Autodesk Inventor part; units mm, degrees
ref_plane "XY Plane" through (0, 0, 0) normal (0, 0, 1) x (1, 0, 0)
sketch "Sketch3" plane through (0, 0, 0) normal (0, 0, 1) x (1, 0, 0)
  circle A0 centre (0, 0) radius 7.62
  dimension "d3" = 15.24
extrude "Extrusion2" add sketch "Sketch3" along normal blind 1.27
sketch "Sketch4" plane through (0, 0, 1.27) normal (0, 0, 1) x (1, 0, 0)
  line L0 (0, 7.5994) -> (6.5813, 3.7997)
  line L1 (6.5813, 3.7997) -> (6.5813, -3.7997)
  line L2 (6.5813, -3.7997) -> (0, -7.5994)
  line L3 (0, -7.5994) -> (-6.5813, -3.7997)
  line L4 (-6.5813, -3.7997) -> (-6.5813, 3.7997)
  line L5 (-6.5813, 3.7997) -> (0, 7.5994)
  point P0 (0, 0)
  point P1 (0, 0)
extrude "Extrusion3" add sketch "Sketch4" along normal blind 18.034
sketch "Sketch5" plane through (0, 0, 19.304) normal (0, 0, 1) x (1, 0, 0)
  circle A0 centre (0, 0) radius 6.35
  dimension "d8" = 12.7
extrude "Extrusion4" add sketch "Sketch5" along normal blind 1.27
sketch "Sketch6" plane through (0, 0, 20.574) normal (0, 0, 1) x (1, 0, 0)
  circle A0 centre (0, 0) radius 6.35
  line L0 (6.5813, 3.7997) -> (6.5813, -3.7997)
  line L1 (6.5813, -3.7997) -> (0, -7.5994)
  line L2 (0, -7.5994) -> (-6.5813, -3.7997)
  line L3 (-6.5813, -3.7997) -> (-6.5813, 3.7997)
  line L4 (-6.5813, 3.7997) -> (0, 7.5994)
  line L5 (0, 7.5994) -> (6.5813, 3.7997)
  circle A1 centre (0, 0) radius 7.62
  line L6 (0, 7.5994) -> (6.5813, 3.7997)
  line L7 (6.35, 3.6662) -> (6.35, -3.6662)
  line L8 (6.35, -3.6662) -> (0, -7.3323)
  line L9 (0, -7.3323) -> (-6.35, -3.6662)
  line L10 (-6.35, -3.6662) -> (-6.35, 3.6662)
  line L11 (-6.35, 3.6662) -> (0, 7.3323)
  line L12 (0, 7.3323) -> (6.35, 3.6662)
  point P0 (3.175, 5.4993)
extrude "Extrusion5" add sketch "Sketch6" along normal blind 1.27 contours A0 | L7 L8 A0 | A0 L12 L7 | A0 L11 L12 | L8 L9 A0 | A0 L10 L11 | L9 L10 A0
sketch "Sketch7" plane through (0, 0, 21.844) normal (0, 0, 1) x (1, 0, 0)
  circle A0 centre (0, 0) radius 3
  dimension "d13" = 6
extrude "Extrusion6" cut sketch "Sketch7" against normal up to next
ref_plane "Work Plane1" through (0, 0, 0) normal (0, 1, 0) x (-1, 0, 0)
ref_plane "Work Plane2" through (0, 0, 0) normal (1, 0, 0) x (0, 1, 0)
properties part number "BaneBots-T40-6mm-Shaft-Adapter"
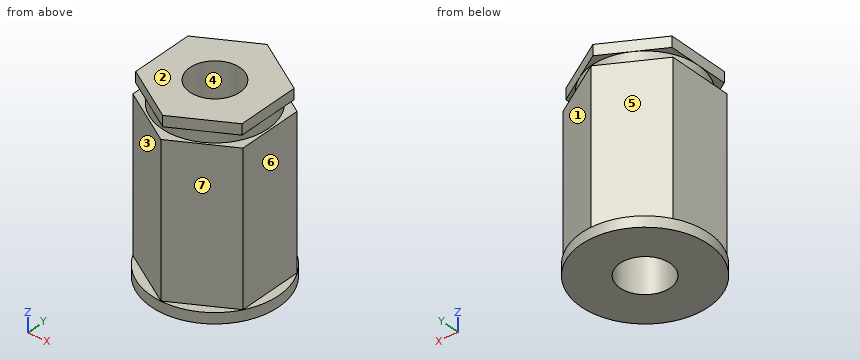
Geometry check sheet. Reference: the model listing, model coordinates, mm. Face numbers are marked on the shaded views. A direction names the side the tool comes from. Give positions to 0.01 mm unless a question says otherwise; leave off trailing zeros. Write each loop counter-clockwise with the first axis right and the second up, starting at its lowest first coordinate (ties: lowest second). Pieces come first, ordered by that corner, then holes. Notation, with made-up numbers: (56.25, 55) -> (78.25, 55) arc R16 ccw to (78.25, 77) -> close; hole circle Ø2 at (-31, 54). An arc over 180 degrees is marked (long way). Use one line per item in the form item = value.
Item 1: Sectioned sample at D-D on y = 5. Enter the section's corners in (x, z).
Results list:
outline = (-5.75, 0) -> (5.75, 0) -> (5.75, 1.27) -> (4.5, 1.27) -> (4.5, 19.3) -> (3.91, 19.3) -> (3.91, 20.57) -> (4.04, 20.57) -> (4.04, 21.84) -> (-4.04, 21.84) -> (-4.04, 20.57) -> (-3.91, 20.57) -> (-3.91, 19.3) -> (-4.5, 19.3) -> (-4.5, 1.27) -> (-5.75, 1.27) -> close
Item 2: Sectioned sample at B-B on y = -1.5. Enter the section's corners in (x, z).
Results list:
outline = (-7.47, 0) -> (-2.6, 0) -> (-2.6, 21.84) -> (-6.35, 21.84) -> (-6.35, 20.57) -> (-6.17, 20.57) -> (-6.17, 19.3) -> (-6.58, 19.3) -> (-6.58, 1.27) -> (-7.47, 1.27) -> close; (2.6, 0) -> (7.47, 0) -> (7.47, 1.27) -> (6.58, 1.27) -> (6.58, 19.3) -> (6.17, 19.3) -> (6.17, 20.57) -> (6.35, 20.57) -> (6.35, 21.84) -> (2.6, 21.84) -> close
Item 3: Access from +Z, -Z, +X, -X, +Y, -Y to the whole of each face (thin tool, end or side, straight path). Record for the marked faces 5, 6 and 7.
Results list:
face_5 = +Z, -X, +Y
face_6 = +Z, +X, +Y, -Y
face_7 = +Z, +X, -Y
Item 4: Sectioned sample at C-C on x = 4.75. Enter the section's corners in (y, z).
Results list:
outline = (-5.96, 0) -> (5.96, 0) -> (5.96, 1.27) -> (4.86, 1.27) -> (4.86, 19.3) -> (4.21, 19.3) -> (4.21, 20.57) -> (4.59, 20.57) -> (4.59, 21.84) -> (-4.59, 21.84) -> (-4.59, 20.57) -> (-4.21, 20.57) -> (-4.21, 19.3) -> (-4.86, 19.3) -> (-4.86, 1.27) -> (-5.96, 1.27) -> close
Item 5: Sectioned sample at A-A on z = 10.75. Enter the section's corners in (x, y), plus the area to 3 significant figures.
Results list:
outline = (-6.58, -3.8) -> (0, -7.6) -> (6.58, -3.8) -> (6.58, 3.8) -> (0, 7.6) -> (-6.58, 3.8) -> close; hole circle Ø6 at (0, 0)
area = 122 mm2
Item 6: Depth check by flat-ended pin: pin 1 Ø0.6 at (y, z) = (-1.5, 21.5) entering from +X; pin 2 Ø1.4 at (y, z) = (1.5, 21) entering from -X; pin 3 Ø1.5 at (x, z) = (1.5, 8) entering from +Y. Enter the tip coordinate at first touch or a pass-through.
Results list:
pin_1 = 6.35
pin_2 = -6.35
pin_3 = 7.17
Item 7: Mould release check, pull along X, two halves, no side actions. Record for the marked faces 1, 2, 3 and 4: released by +X, released by -X, zero draft, split by the parting line, or undercut.
Results list:
face_1 = released by +X
face_2 = zero draft
face_3 = released by -X
face_4 = undercut
Item 8: Scan lines: line 1 (Z direction, x = 0.75, y = 6.5); line 2 (Z direction, x = -5.25, y = 4.5); line 3 (X direction, y = 1.25, z = 3.5). Record each from-to range of solid material in increasing order.
Results list:
line_1 = 0 to 19.3, 20.57 to 21.84
line_2 = 0 to 19.3
line_3 = -6.58 to -2.73, 2.73 to 6.58
